Job drawing, mm, ordinate dimensions from the low corner. One solid piece. A direction names the side the tool comes from. Give positions to 0.01 mm unless a question says otherwise; leave off trailing zeros. Write each loop counter-clockwise with the first axis right and the second up, starting at its lowest first coordinate (ties: lowest second). Pieces come first, ordered by that corner, then holes. Notation, with made-up numbers: (-19, 89) - (5, 89) arc R11 cw to (5, 97) - close; hole circle Ø11 at (44.5, -39). An arc over 180 degrees is marked (long way). Answer as a JSON object with one key per item and string values.
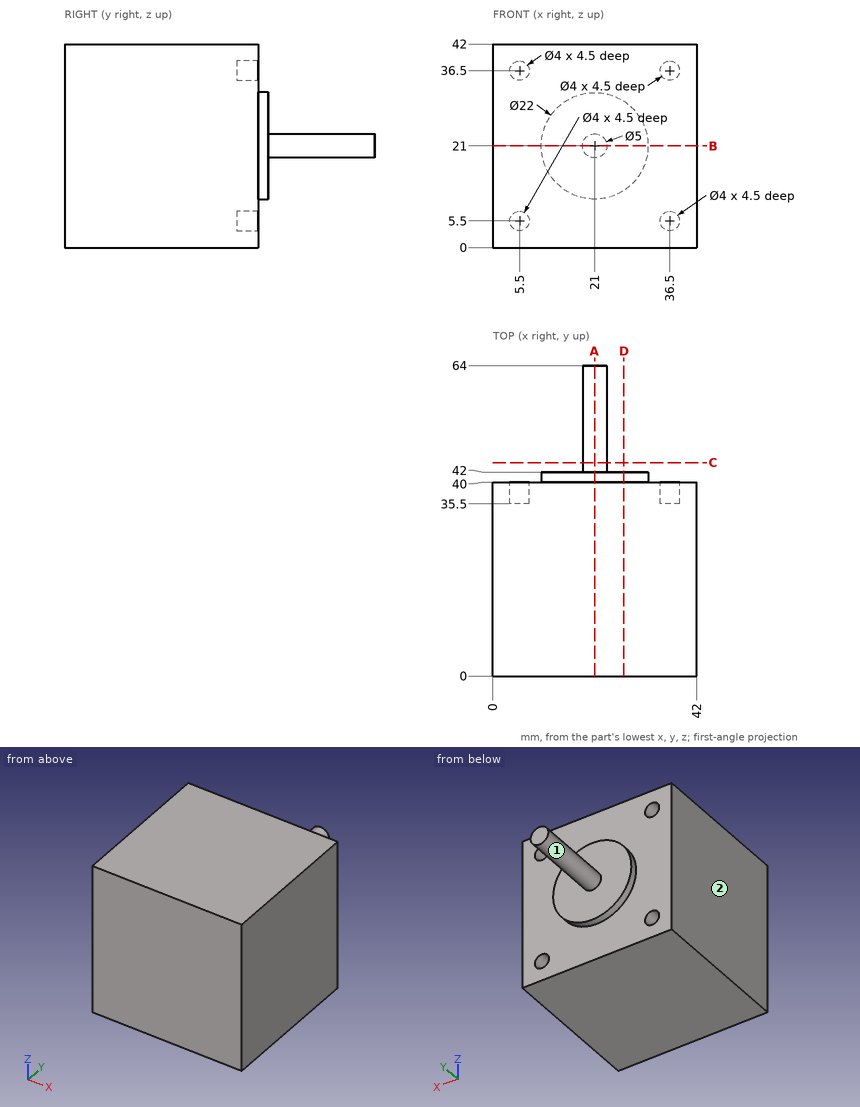
Item 1: Cut at A-A (x = 21). Give the cut face in (y, z).
Entries:
{"outline": "(0, 0) - (40, 0) - (40, 10) - (42, 10) - (42, 18.5) - (64, 18.5) - (64, 23.5) - (42, 23.5) - (42, 32) - (40, 32) - (40, 42) - (0, 42) - close"}
Item 2: Cut at D-D (x = 27). Give the cut face in (y, z).
Entries:
{"outline": "(0, 0) - (40, 0) - (40, 11.78) - (42, 11.78) - (42, 30.22) - (40, 30.22) - (40, 42) - (0, 42) - close"}
Item 3: Which spindle directions (+Z, -Z, +X, -X, +Y, -Y) get a long thin tool onto all of the face, cutting with end or side? Do the marked faces 1 and 2. Say none if no direction does.
Entries:
{"face 1": "+Y", "face 2": "+Z, -Z, -X, +Y, -Y"}
Item 4: Cut at B-B (z = 21). Give the cut face in (x, y), and give its area (3 significant figures).
Entries:
{"outline": "(0, 0) - (42, 0) - (42, 40) - (32, 40) - (32, 42) - (23.5, 42) - (23.5, 64) - (18.5, 64) - (18.5, 42) - (10, 42) - (10, 40) - (0, 40) - close", "area": "1,830 mm2"}
Item 5: Probe line 1 (X direction, y = 39.05, z = 36.5); line 2 (Z direction, x = 5, y = 38). List the from-to ranges inside material, lowest first. Write a range as from..to.
Entries:
{"line 1": "0..3.5, 7.5..34.5, 38.5..42", "line 2": "0..3.56, 7.44..34.56, 38.44..42"}
Item 6: Cut at C-C (y = 44). Give the cut face in (x, z), and give its area (3 significant figures).
Entries:
{"outline": "circle Ø5 at (21, 21)", "area": "19.6 mm2"}
Item 7: Flat gauge pins, fed straight in: P1, Ø3, axis at x = 6.5, z = 6.5, coming from the +Y side; P2, Ø2.5, axis at x = 5.5, z = 36.5, coming from the +Y side; P3, Ø2, axis at y = 47, z = 21, coming from the -X side. Where does each tip first touch, or does it go through?
Entries:
{"P1": "y = 40", "P2": "y = 35.5", "P3": "x = 18.5"}
